Autodesk Inventor part; units mm, degrees
ref_plane "Work Plane3" through (0, 0, 15.875) normal (0, 0, 1) x (1, 0, 0)
ref_plane "Work Plane4" through (15.875, 0, 0) normal (1, 0, 0) x (0, 1, 0)
ref_plane "YZ Plane" through (0, 0, 0) normal (1, 0, 0) x (0, 1, 0)
sketch "Sketch1" plane through (0, 0, 0) normal (0, 1, 0) x (-1, 0, 0)
  circle A0 centre (0, 0) radius 15.875
  dimension "d0" = 31.75
extrude "Extrusion1" add sketch "Sketch1" along normal blind 550
sketch "Sketch7" plane through (0, 550, 0) normal (0, 1, 0) x (1, 0, 0)
  circle A0 centre (0, 0) radius 15.075
  dimension "d23" = 30.15
extrude "Extrusion3" cut sketch "Sketch7" against normal through all
sketch "Sketch8" plane through (0, 0, 0) normal (0, -1, 0) x (1, 0, 0)
  circle A0 centre (0, 0) radius 15.875
  point P0 (0, 15.875)
ref_plane "Work Plane3" through (0, 0, 15.875) normal (0, 0, 1) x (1, 0, 0)
sketch "Sketch9" plane through (0, 0, 15.875) normal (0, 0, 1) x (1, 0, 0)
  arc A0 (15.075, 5) -> (-15.075, 5) centre (0, 5) ccw
  line L0 (-15.075, 5) -> (-15.075, 0)
  line L1 (15.875, 0) -> (-15.875, 0)
  line L2 (15.075, 5) -> (15.075, 0)
  point P0 (0, 0)
  dimension "d26" = 5
  dimension "d27" = 30.15
extrude "Extrusion4" cut sketch "Sketch9" against normal through all
sketch "Sketch10" plane through (0, 0, 0) normal (0, -1, 0) x (1, 0, 0)
  circle A0 centre (0, 0) radius 15.875
  point P0 (15.875, 0)
ref_plane "Work Plane4" through (15.875, 0, 0) normal (1, 0, 0) x (0, 1, 0)
sketch "Sketch11" plane through (15.875, 0, 0) normal (1, 0, 0) x (0, 1, 0)
  line L0 (0, -4.9759) -> (0, 4.9759)
  point P0 (0, 0)
  point P1 (5, 0)
  point P2 (0, 0)
  dimension "d30" = 5
hole "Hole3" at (15.875, 5, 0) direction (-1, 0, 0) diameter 3.4587 end through all
equation "\"d36\" = Thickness"
equation "\"BendRadius\" = Thickness"
equation "\"BendReliefWidth\" = Thickness"
equation "\"BendReliefDepth\" = 0.5 * Thickness"
equation "\"CornerReliefSize\" = 4 * Thickness"
equation "\"MinimumRemnant\" = 2 * Thickness"
equation "\"TransitionRadius\" = BendRadius"
equation "\"JacobiRadiusSize\" = BendRadius"
equation "\"GapSize\" = Thickness"
properties part number "Output link body_ final"
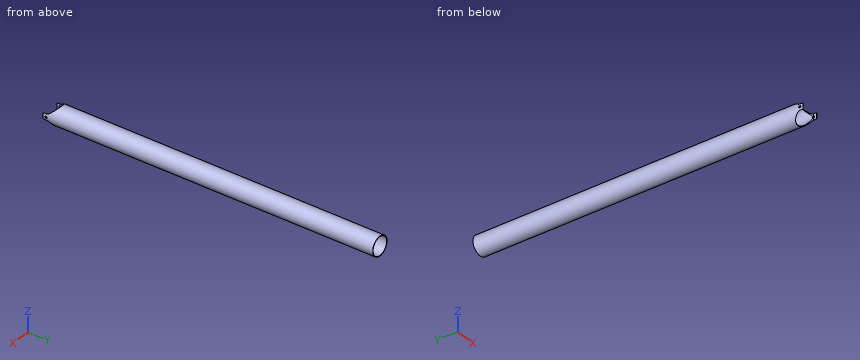
Part model, mm, in its own coordinate system. Coordinates: 2 decimals unless noted, no trailing zeros. Loops run counter-clockwise (first coordinate to the right, second up) from the corner with the lowest first, then second, coordinate; pieces in that order, holes last. Notation, with made-up numbers: M -13.75,66 L 25.25,66 A23 cw 25.25,96 Z; hole C 81.5,-21.5 d1. An arc over 180 degrees is marked long. Use a Markdown table: item, result. Add a question column.
Q1. Pin check, flat tips, straight feed: P1, Ø2, axis at x = 7, y = 150, coming from the -Z side; P2, Ø1.5, axis at y = 253, z = -10.5, coming from the -X side; P3, Ø2, axis at y = 252, z = -12, coming from the +X side. Stop position of each tip, or through.
Q2. Cut at C-C (y = 118). Write the cut outline in (x, z) (3 decimals), and give its area (3 significant figures).
Q3. Cut at A-A (x = 0). Write the cut outline in (y, z) (3 decimals), and give its area (3 significant figures).
Q4. Probe L1, parallel to Z at x = -1, y = 411; L2, parallel to Z at x = 0, y = 288 (3 decimals). List the from-to ranges inside material, lowest first.
Q5. Cut at B-B (z = -10.5). Write the cut outline in (x, y) (3 decimals).
Worked out:
| question | item | result |
|---|---|---|
| 1 | P1 | stops at z = -14.7 |
| 1 | P2 | stops at x = -12.53 |
| 1 | P3 | stops at x = 11.45 |
| 2 | outline | C 0,0 d31.75; hole C 0,0 d30.15 |
| 2 | area | 77.8 mm2 |
| 3 | outline | M 20.075,-15.875 L 550,-15.875 L 550,-15.075 L 20.075,-15.075 Z; M 20.075,15.075 L 550,15.075 L 550,15.875 L 20.075,15.875 Z |
| 3 | area | 848 mm2 |
| 4 | L1 | z = -15.84 to -15.04, 15.04 to 15.84 |
| 4 | L2 | z = -15.875 to -15.075, 15.075 to 15.875 |
| 5 | outline | M -11.907,14.246 A15.075 cw -10.817,15.5 L -10.817,550 L -11.907,550 Z; M 10.817,15.5 A15.075 cw 11.907,14.246 L 11.907,550 L 10.817,550 Z |
